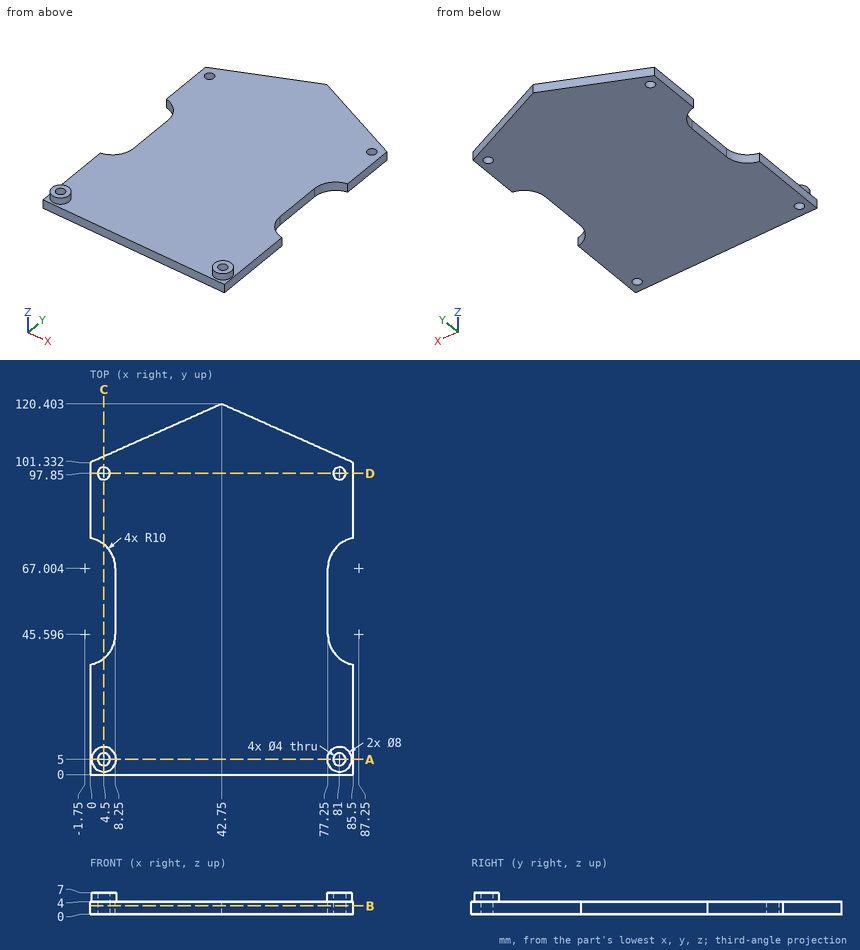
Part print with two shaded views. Sizes in mm from the minimum x, y, z corner. Coordinates: 2 decimals unless noted, no trailing zeros. Write each loop counter-clockwise with the first axis right and the second up, starting at its lowest first coordinate (ties: lowest second). Pieces come first, ordered by that corner, then holes. Notation, with made-up numbers: (41.5, 12.25) -> (62.5, 12.25) arc R21 cw to (62.5, 29.25) -> close; hole circle Ø6 at (-25.75, 63.5). An arc over 180 degrees is marked (long way). Return JSON: item names as keys, results as strings. Group by question number.
Q1. Drill centre lines: line 1 (Y direction, x = 81, z = 5.5); line 2 (Y direction, x = 4.5, z = 2.6); line 3 (Z direction, x = 39, y = 8). Where is each one in solid material? Low to high.
Q2. Cut at D-D, the plane y = 97.85. Give the cut face in (x, z), then the cut area to 3 significant figures.
Q3. Cut at C-C, the plane x = 4.5. Give the cut face in (y, z), then the cut area to 3 significant figures.
Q4. Cut at B-B, the plane z = 2.75. Give the cut face in (x, y).
Q5. Cut at A-A, the plane y = 5. Give the cut face in (x, z), then the cut area to 3 significant figures.
Q6. Flat gauge pins, fed straight in: pin 1 (1.2 mm diameter, centred on y = 53.5, z = 1.5, fed in from +X); pin 2 (4 mm diameter, centred on y = 42.5, z = 4, fed in from +X) (1 decimal); pin 3 (3.5 mm diameter, centred on x = 81, y = 97.85, fed in from +Z); pin 4 (2 mm diameter, centred on y = 59, z = 2, fed in from -X). Where does each tip first touch, or does it go through?
Returned:
{
 "1": {"line 1": "y = 1 to 3, 7 to 9", "line 2": "y = 0 to 3, 7 to 37.79, 74.81 to 95.85, 99.85 to 103.34", "line 3": "z = 0 to 4"},
 "2": {"outline": "(0, 0) -> (2.5, 0) -> (2.5, 4) -> (0, 4) -> close; (6.5, 0) -> (79, 0) -> (79, 4) -> (6.5, 4) -> close; (83, 0) -> (85.5, 0) -> (85.5, 4) -> (83, 4) -> close", "area": "310 mm2"},
 "3": {"outline": "(0, 0) -> (3, 0) -> (3, 7) -> (1, 7) -> (1, 4) -> (0, 4) -> close; (7, 0) -> (37.79, 0) -> (37.79, 4) -> (9, 4) -> (9, 7) -> (7, 7) -> close; (74.81, 0) -> (95.85, 0) -> (95.85, 4) -> (74.81, 4) -> close; (99.85, 0) -> (103.34, 0) -> (103.34, 4) -> (99.85, 4) -> close", "area": "245 mm2"},
 "4": {"outline": "(0, 0) -> (85.5, 0) -> (85.5, 35.75) arc R10 cw to (77.25, 45.6) -> (77.25, 67) arc R10 cw to (85.5, 76.85) -> (85.5, 101.33) -> (42.75, 120.4) -> (0, 101.33) -> (0, 76.85) arc R10 cw to (8.25, 67) -> (8.25, 45.6) arc R10 cw to (0, 35.75) -> close; hole circle Ø4 at (4.5, 5); hole circle Ø4 at (4.5, 97.85); hole circle Ø4 at (81, 5); hole circle Ø4 at (81, 97.85)"},
 "5": {"outline": "(0, 0) -> (2.5, 0) -> (2.5, 7) -> (0.5, 7) -> (0.5, 4) -> (0, 4) -> close; (6.5, 0) -> (79, 0) -> (79, 7) -> (77, 7) -> (77, 4) -> (8.5, 4) -> (8.5, 7) -> (6.5, 7) -> close; (83, 0) -> (85.5, 0) -> (85.5, 4) -> (85, 4) -> (85, 7) -> (83, 7) -> close", "area": "334 mm2"},
 "6": {"pin 1": "stops at x = 77.25", "pin 2": "stops at x = 78.6", "pin 3": "passes through", "pin 4": "stops at x = 8.25"}
}
